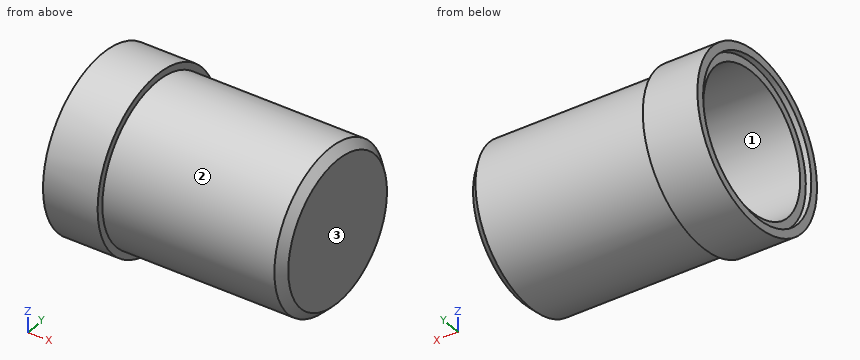
```python
from build123d import *

# Parameters (mm, degrees)
ESBO_O2_R             = 2.848867015
CORTE_EXTRUS_O1_DEPTH = 0.2


with BuildPart() as part:
    # Esboço1 → Revolução1 (revolve)
    with BuildSketch(Plane.XY, mode=Mode.PRIVATE) as revolu_o1_sk:
        Polygon((8.3, 2.9), (8.6, 2.6), (8.6, 2.55), (8.6, 0), (8.45, 0), (8.45, 2.55), (0, 2.55), (0, 3.15), (2, 3.15), (2, 2.9), align=None)
    revolve(revolu_o1_sk.sketch.rotate(Axis((0, 0, 0), (1, 0, 0)), 180), axis=Axis((0, 0, 0), (1, 0, 0)))

    # Esboço2 → Corte-extrusão1 (cut)
    with BuildSketch(Plane(origin=(0, 0, 0), x_dir=(0, 0, -1), z_dir=(1, 0, 0))):
        Circle(ESBO_O2_R)
    extrude(amount=CORTE_EXTRUS_O1_DEPTH, mode=Mode.SUBTRACT)


solid = part.part
```
Geometry: final body of the model. Coordinates: model frame, mm. Face numbers are marked on the shaded views. Coordinates: 2 decimals unless noted, no trailing zeros. Order: outer loops, then holes, each group sorted by start corner. A loop starts at its lowest first (then second) coordinate and runs counter-clockwise, first axis right, second up. Notation, with made-up numbers: (-22, 32) -> (34, 32) arc R11 ccw to (34, 40) -> close; hole circle Ø4 at (16, 4.5). An arc over 180 degrees is marked (long way). Write item = value, one per line.
(1) Cut plane D-D on x = 7. Return loops of the section in (y, z).
Solved:
outline = circle Ø5.8 at (0, 0); hole circle Ø5.1 at (0, 0)
(2) Pull-direction query (Z, two-part tool) for the marked faces 1, 2 and 3; classes: pulls with the +Z half, pulls with the -Z half, needs draft (parallel to the pull), parting line crosses it, or undercut.
Solved:
face_1 = undercut
face_2 = parting line crosses it
face_3 = needs draft
(3) Line query: line 1 (Z direction, x = 4.25, y = 0); line 2 (Z direction, x = 1, y = -1.5); line 3 (X direction, y = 0.25, z = 3). Output: solid intervals per line, ascending.
Solved:
line_1 = -2.9 to -2.55, 2.55 to 2.9
line_2 = -2.77 to -2.06, 2.06 to 2.77
line_3 = 0 to 2
(4) Cut plane C-C on x = 1.5. Return loops of the section in (y, z).
Solved:
outline = circle Ø6.3 at (0, 0); hole circle Ø5.1 at (0, 0)
(5) Pin query (flat end, axial travel): pin 1 Ø3.5 at (y, z) = (0, 0) entering from -X; pin 2 Ø1 at (x, z) = (6, 1) entering from +Y; pin 3 Ø2 at (x, y) = (4, 1.5) entering from -Z. Return the tip coordinate at first contact, or that it passes through.
Solved:
pin_1 = 8.45
pin_2 = 2.86
pin_3 = -2.86
(6) Cut plane A-A on y = 0. Return loops of the section in (x, z), plus the area to 3 significant figures.
Solved:
outline = (0, -3.15) -> (2, -3.15) -> (2, -2.9) -> (8.3, -2.9) -> (8.6, -2.6) -> (8.6, 2.6) -> (8.3, 2.9) -> (2, 2.9) -> (2, 3.15) -> (0, 3.15) -> (0, 2.85) -> (0.2, 2.85) -> (0.2, 2.55) -> (8.45, 2.55) -> (8.45, -2.55) -> (0.2, -2.55) -> (0.2, -2.85) -> (0, -2.85) -> close
area = 7.58 mm²
